Design review of the part built by this model. Coordinates are the model's own, in mm. A direction names the side the tool comes from. Round coordinates to 2 decimals unless told otherwise and drop trailing zeros. Loops run counter-clockwise (first coordinate to the right, second up) from the corner with the lowest first, then second, coordinate; pieces in that order, holes last. Notation, with made-up numbers: (-0.75, -8.75) -> (8.25, -8.75) arc R16 ccw to (8.25, 7.25) -> close; hole circle Ø4 at (89, -2.5). An arc over 180 degrees is marked (long way). Answer as CSV lines item,"result". Start each with the question number.
Autodesk Inventor part; units mm, degrees
ref_plane "YZ Plane" through (0, 0, 0) normal (1, 0, 0) x (0, 1, 0)
ref_plane "XZ Plane" through (0, 0, 0) normal (0, 1, 0) x (-1, 0, 0)
ref_plane "XY Plane" through (0, 0, 0) normal (0, 0, 1) x (1, 0, 0)
sketch "Sketch1" plane through (0, 0, 0) normal (0, 0, 1) x (1, 0, 0)
  line L0 (0, 0) -> (0, 27.8)
  line L1 (0, 27.8) -> (58.6, 27.8)
  line L2 (58.6, 27.8) -> (58.6, 0)
  line L3 (58.6, 0) -> (0, 0)
  line L4 (9, 23.8) -> (49.6, 23.8)
  line L5 (49.6, 23.8) -> (49.6, 4)
  line L6 (49.6, 4) -> (9, 4)
  line L7 (9, 4) -> (9, 23.8)
  point P0 (29.3, 23.8)
  point P1 (29.3, 27.8)
  point P2 (29.3, 4)
  point P3 (58.6, 13.9)
  point P4 (49.6, 13.9)
  dimension "d0" = 58.6
  dimension "d1" = 27.8
  dimension "d2" = 40.6
  dimension "d3" = 19.8
  dimension "d4" = 4
  dimension "d5" = 4
  dimension "d6" = 9
  dimension "d7" = 9
extrude "Extrusion1" add sketch "Sketch1" along normal blind 22
fillet "Fillet1" radius 2 4 edges at (0, 0, 11) (0, 27.8, 11) (58.6, 27.8, 11) (58.6, 0, 11)
fillet "Fillet2" radius 1 16 edges at (0, 13.9, 22) (0.5858, 27.2142, 22) (29.3, 27.8, 22) (58.0142, 27.2142, 22) (58.6, 13.9, 22) (58.0142, 0.5858, 22) (29.3, 0, 22) (0.5858, 0.5858, 22) (29.3, 0, 0) (58.0142, 0.5858, 0) (58.6, 13.9, 0) (58.0142, 27.2142, 0) (29.3, 27.8, 0) (0.5858, 27.2142, 0) (0, 13.9, 0) (0.5858, 0.5858, 0)
sketch "Sketch2" plane through (0, 0, 0) normal (0, 0, -1) x (-1, 0, 0)
  point P0 (0, 0)
sketch "Sketch3" plane through (0, 0, 0) normal (0, 0, -1) x (-1, 0, 0)
  point P0 (0, 0)
properties part number "servo_to_links"
Q1. For pin 1 Ø5 at (y, z) = (13, 4) entering from -X, flat-tipped, find the tip position at first contact; note if it passes through.
Q2. Add section B-B, the plane y = 15.75. Give the boundary of the cut face in (x, z).
Q3. Mouldability with a two-part tool opening along Y and no side actions: class faces 1 (the flat face through (49.6, 14, 11)), 2 (the cylindrical face through (0.57, 0.6, 11.14)), 3 (the flat face through (58.6, 14, 11)) as pulls with the +Y half, pulls with the -Y half, needs draft (parallel to the pull), parting line crosses it, or undercut.
Q4. Machinability: for faces 4 (the flat face through (29, 3, 22)), 5 (the flat face through (29, 23.8, 11)), which of the approach directions +Z, -Z, +X, -X, +Y, -Y give a long, thin tool a straight path to every point of the face, cutting with its end or side? Answer none if there is none.
Q5. Add section C-C, the plane z = 17.5. Give the boundary of the cut face in (x, y).
Q6. To check wall thickness, follow probe 1 along X at (y, z) = (14, 11.75); probe 2 along Y at (x, z) = (19.5, 8.75). State the ranges of each line that lie inside material, in increasing order. Write a range as from..to.
Q7. Add section A-A, the plane x = 46. Give the boundary of the cut face in (y, z).
Worked answers:
1,pin 1,"stops at x = 0"
2,outline,"(0, 1) arc R1 ccw to (1, 0) -> (9, 0) -> (9, 22) -> (1, 22) arc R1 ccw to (0, 21) -> close; (49.6, 0) -> (57.6, 0) arc R1 ccw to (58.6, 1) -> (58.6, 21) arc R1 ccw to (57.6, 22) -> (49.6, 22) -> close"
3,face 1,"undercut"
3,face 2,"pulls with the -Y half"
3,face 3,"needs draft"
4,face 4,"+Z, +X, -X, +Y, -Y"
4,face 5,"+Z, -Z"
5,outline,"(0, 2) arc R2 ccw to (2, 0) -> (56.6, 0) arc R2 ccw to (58.6, 2) -> (58.6, 25.8) arc R2 ccw to (56.6, 27.8) -> (2, 27.8) arc R2 ccw to (0, 25.8) -> close; hole (9, 4) -> (49.6, 4) -> (49.6, 23.8) -> (9, 23.8) -> close"
6,probe 1,"x = 0..9, 49.6..58.6"
6,probe 2,"y = 0..4, 23.8..27.8"
7,outline,"(0, 1) arc R1 ccw to (1, 0) -> (4, 0) -> (4, 22) -> (1, 22) arc R1 ccw to (0, 21) -> close; (23.8, 0) -> (26.8, 0) arc R1 ccw to (27.8, 1) -> (27.8, 21) arc R1 ccw to (26.8, 22) -> (23.8, 22) -> close"
